```python
from build123d import *

# Parameters (mm, degrees)
SKETCH1_R           = 52.5
BOSS_EXTRUDE1_DEPTH = 9
SKETCH2_R           = 12.5
CUT_EXTRUDE1_DEPTH  = 75.789705174
SKETCH3_R           = 5.677743223
CUT_EXTRUDE2_DEPTH  = 8.396654
CIRPATTERN1_START   = 0.603346211
CIRPATTERN1_DEPTH   = 8.396653789


# Read off the part's stored shape, not the designer's step: CirPattern1
with BuildPart() as part:
    # Sketch1 → Boss-Extrude1 (new body)
    with BuildSketch(Plane(origin=(0, 0, 0), x_dir=(1, 0, 0), z_dir=(0, 1, 0))):
        with Locations(Location((0, 0, 0), (0, 0, 270))):
            Circle(SKETCH1_R)
    extrude(amount=BOSS_EXTRUDE1_DEPTH)

    # Sketch2 → Cut-Extrude1 (cut, through all)
    with BuildSketch(Plane(origin=(0, 0, 0), x_dir=(1, 0, 0), z_dir=(0, 1, 0))):
        with Locations(Location((0, 0, 0), (0, 0, 270))):
            Circle(SKETCH2_R)
    extrude(amount=CUT_EXTRUDE1_DEPTH, mode=Mode.SUBTRACT)

    # Sketch3 → Cut-Extrude2 (cut)
    with BuildSketch(Plane(origin=(0, 9, 0), x_dir=(1, 0, 0), z_dir=(0, 1, 0))):
        with Locations((-12.911355312, 0)):
            Circle(SKETCH3_R)
    extrude(amount=-CUT_EXTRUDE2_DEPTH, mode=Mode.SUBTRACT)

    # CirPattern1 outline → CirPattern1 (cut)
    with BuildSketch(Plane(origin=(0, 0, 0), x_dir=(1, 0, 0), z_dir=(0, 1, 0)).offset(CIRPATTERN1_START)):
        with BuildLine():
            ThreePointArc((-5.431733493, 11.258164649), (0, 12.5), (5.431733493, 11.258164649))
            ThreePointArc((5.431733493, 11.258164649), (0, 18.589098535), (-5.431733493, 11.258164649))
        make_face()
        with BuildLine():
            ThreePointArc((11.258164649, -5.431733493), (18.589098535, 0), (11.258164649, 5.431733493))
            ThreePointArc((11.258164649, 5.431733493), (12.5, 0), (11.258164649, -5.431733493))
        make_face()
        with BuildLine():
            ThreePointArc((5.431733493, -11.258164649), (0, -12.5), (-5.431733493, -11.258164649))
            ThreePointArc((-5.431733493, -11.258164649), (0, -18.589098535), (5.431733493, -11.258164649))
        make_face()
    extrude(amount=CIRPATTERN1_DEPTH, mode=Mode.SUBTRACT)


solid = part.part
```
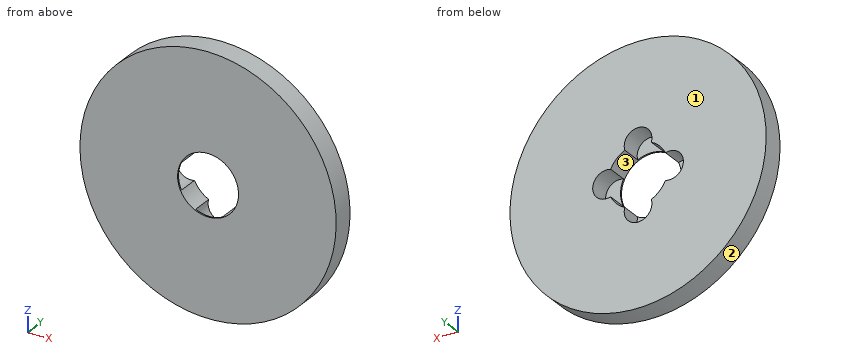
Design review of the part built by this model. Coordinates are the model's own, in mm. Face numbers are marked on the shaded views. Give positions to 0.01 mm unless a question says otherwise; leave off trailing zeros. Order: outer loops, then holes, each group sorted by start corner. A loop starts at its lowest first (then second) coordinate and runs counter-clockwise, first axis right, second up. Notation, with made-up numbers: (52, 87.25) - (109, 87.25) arc R30 ccw to (109, 123.25) - close; hole circle Ø8 at (-37.5, -7). An arc over 180 degrees is marked (long way). Use a Markdown table: item, result. Add a question column.
(1) Clearance check with flat-ended pins moving along their axes: P1, Ø9, axis at x = 12.91, z = 0, coming from the +Y side; P2, Ø1, axis at x = 20, y = 7.5, coming from the +Z side; P3, Ø2, axis at x = -30, y = 2.5, coming from the +Z side. State where each tip first meets the part, or that it passes through.
(2) Add section B-B on z = 0. Give the boundary of the cut face in (x, y), then the cut area to 3 significant figures.
(3) Add section A-A on x = 0. Give the boundary of the cut face in (y, z), then the cut area to 3 significant figures.
(4) Wall thickness on probe 1 along X at (y, z) = (8, 0); probe 2 along X at (y, z) = (8.25, 1.5); probe 3 along Z at (x, y) = (15, 3.25): over which ranges is each line inside the solid? List them lowest first. Write a range as [from, to].
(5) Mouldability with a two-part tool opening along X and no side actions: class the marked faces 1, 2 and 3 as +X half, -X half, draft (parallel to the pull), parting line (faces both ways), or undercut.
(6) Add section C-C on y = 2.5. Give the boundary of the cut face in (x, z).
(7) Add section D-D on x = 17. Give the boundary of the cut face in (y, z).
Report:
| question | item | result |
|---|---|---|
| 1 | P1 | stops at y = 0.6 |
| 1 | P2 | stops at z = 48.74 |
| 1 | P3 | stops at z = 43.76 |
| 2 | outline | (-52.5, 0) - (-12.5, 0) - (-12.5, 0.6) - (-18.59, 0.6) - (-18.59, 9) - (-52.5, 9) - close; (12.5, 0) - (52.5, 0) - (52.5, 9) - (18.59, 9) - (18.59, 0.6) - (12.5, 0.6) - close |
| 2 | area | 618 mm² |
| 3 | outline | (0, -52.5) - (9, -52.5) - (9, -18.59) - (0.6, -18.59) - (0.6, -12.5) - (0, -12.5) - close; (0, 12.5) - (0.6, 12.5) - (0.6, 18.59) - (9, 18.59) - (9, 52.5) - (0, 52.5) - close |
| 3 | area | 618 mm² |
| 4 | probe 1 | x = [-52.5, -18.59], [18.59, 52.5] |
| 4 | probe 2 | x = [-52.48, -18.39], [18.39, 52.48] |
| 4 | probe 3 | z = [-50.31, -5.28], [5.28, 50.31] |
| 5 | face 1 | draft |
| 5 | face 2 | parting line |
| 5 | face 3 | undercut |
| 6 | outline | circle Ø105 at (0, 0); hole (-11.26, -5.43) arc R12.5 ccw to (-5.43, -11.26) arc R5.68 ccw (long way) to (5.43, -11.26) arc R12.5 ccw to (11.26, -5.43) arc R5.68 ccw (long way) to (11.26, 5.43) arc R12.5 ccw to (5.43, 11.26) arc R5.68 ccw (long way) to (-5.43, 11.26) arc R12.5 ccw to (-11.26, 5.43) arc R5.68 ccw (long way) to start |
| 7 | outline | (0, -49.67) - (9, -49.67) - (9, -3.94) - (0.6, -3.94) - (0.6, 3.94) - (9, 3.94) - (9, 49.67) - (0, 49.67) - close |
